Geometry check sheet. Reference: drawing and pictorial views, mm from the part's lowest x, y, z. A direction names the side the tool comes from. Coordinates: 2 decimals unless noted, no trailing zeros. Write each loop counter-clockwise with the first axis right and the second up, starting at its lowest first coordinate (ties: lowest second). Pieces come first, ordered by that corner, then holes. Notation, with made-up numbers: M 47.25,64.25 L 79.25,64.25 A17 cw 79.25,84.25 Z; hole C 56,39 d1. An arc over 180 degrees is marked long. One line per item, written item: value.
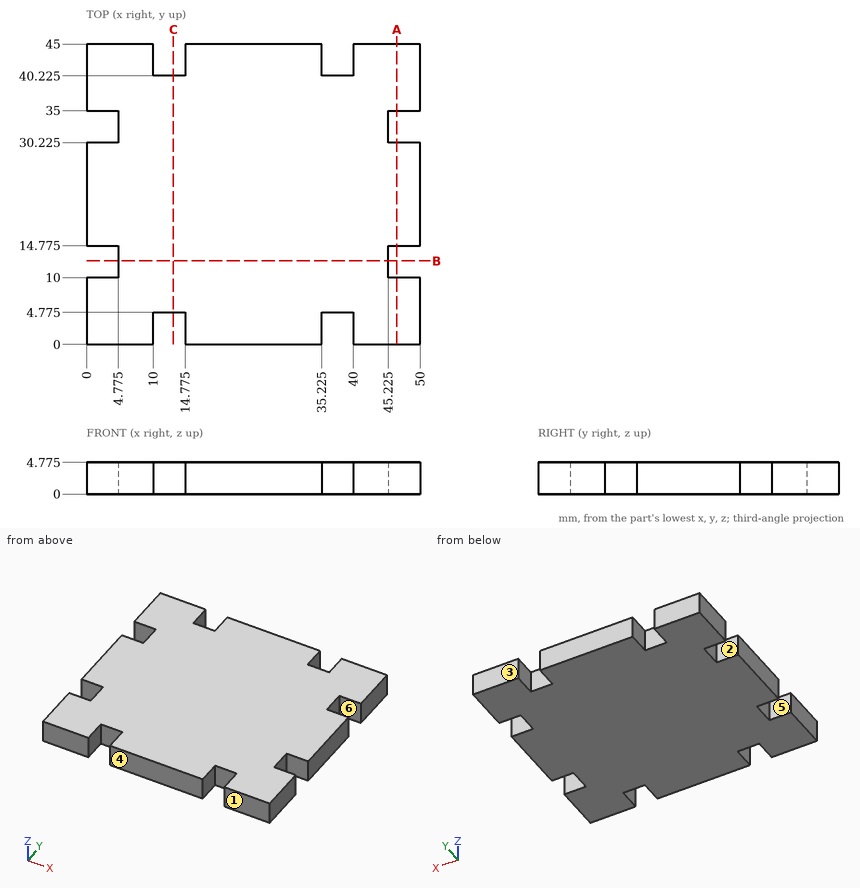
Item 1: Cross-section at B-B, the plane y = 12.5. Enter the section's corners in (x, z) (1 decimal), and give its area (3 significant figures).
The answers:
outline: M 4.8,0 L 45.2,0 L 45.2,4.8 L 4.8,4.8 Z
area: 193 mm²
Item 2: Draft check along Y on the marked faces 1, 2 and 3. Enter one of: released by +Y, released by -Y, zero draft, split by the parting line, or undercut.
The answers:
face 1: released by -Y
face 2: undercut
face 3: released by +Y
Item 3: Scan lines: line 1 (X direction, y = 4, z = 4.2) (1 decimal); line 2 (Y direction, x = 3, z = 1.5) (1 decimal); line 3 (X direction, y = 34, z = 0.2) (1 decimal). Record each from-to range of solid material in increasing order.
The answers:
line 1: x = 0 to 10, 14.8 to 35.2, 40 to 50
line 2: y = 0 to 10, 14.8 to 30.2, 35 to 45
line 3: x = 4.8 to 45.2
Item 4: Cross-section at A-A, the plane x = 46.5. Enter the section's corners in (y, z) (1 decimal), and give its area (3 significant figures).
The answers:
outline: M 0,0 L 10,0 L 10,4.8 L 0,4.8 Z; M 14.8,0 L 30.2,0 L 30.2,4.8 L 14.8,4.8 Z; M 35,0 L 45,0 L 45,4.8 L 35,4.8 Z
area: 169 mm²
Item 5: Cross-section at C-C, the plane x = 13. Enter the section's corners in (y, z) (1 decimal).
The answers:
outline: M 4.8,0 L 40.2,0 L 40.2,4.8 L 4.8,4.8 Z
Item 6: Go/stop test with a flat-tipped pin: P1, Ø1.4, axis at x = 37, z = 3, coming from the -Y side (3 decimals). Record where the tip stops, or that it passes through.
The answers:
P1: stops at y = 4.775
Item 7: Access from +Z, -Z, +X, -X, +Y, -Y to the whole of each face (thin tool, end or side, straight path). Record for the marked faces 4, 5 and 6.
The answers:
face 4: +Z, -Z, +X, -X, -Y
face 5: +Z, -Z, -X
face 6: +Z, -Z, +X
